```python
from build123d import *

# Parameters (mm, degrees)
F0_W     = 270
F0_H     = 32
F0_W_2   = 268
F0_H_2   = 30
F1_DEPTH = 210
F2_R     = 22.9
F3_DEPTH = 1
F4_R     = 1.5
F5_R     = 1


with BuildPart() as f1:
    # F0 (on Right) → F1 (new body)
    with BuildSketch(Plane.YZ):
        with Locations((135, -16)):
            Rectangle(F0_W, F0_H)
        with Locations((135, -16)):
            Rectangle(F0_W_2, F0_H_2, mode=Mode.SUBTRACT)
    extrude(amount=F1_DEPTH)

    # F2 (on face) → F3 (cut, through all)
    with BuildSketch(Plane.XY):
        with Locations((27.8, 29.6)):
            Circle(F2_R)
        with Locations((27.8, 82.6)):
            Circle(F2_R)
        with Locations((27.8, 135.6)):
            Circle(F2_R)
        with Locations((27.8, 188.6)):
            Circle(F2_R)
        with Locations((27.8, 241.6)):
            Circle(F2_R)
        with Locations((78.8, 29.6)):
            Circle(F2_R)
        with Locations((78.8, 82.6)):
            Circle(F2_R)
        with Locations((78.8, 135.6)):
            Circle(F2_R)
        with Locations((78.8, 188.6)):
            Circle(F2_R)
        with Locations((78.8, 241.6)):
            Circle(F2_R)
        with Locations((129.8, 29.6)):
            Circle(F2_R)
        with Locations((129.8, 82.6)):
            Circle(F2_R)
        with Locations((129.8, 135.6)):
            Circle(F2_R)
        with Locations((129.8, 188.6)):
            Circle(F2_R)
        with Locations((129.8, 241.6)):
            Circle(F2_R)
        with Locations((180.8, 29.6)):
            Circle(F2_R)
        with Locations((180.8, 82.6)):
            Circle(F2_R)
        with Locations((180.8, 135.6)):
            Circle(F2_R)
        with Locations((180.8, 188.6)):
            Circle(F2_R)
        with Locations((180.8, 241.6)):
            Circle(F2_R)
    extrude(amount=-F3_DEPTH, mode=Mode.SUBTRACT)

    # F4
    f4_edges = [f1.edges().sort_by_distance(p)[0] for p in [
        (105, 270, 0),
        (105, 270, -32),
        (105, 0, -32),
        (105, 0, 0),
    ]]
    fillet(f4_edges, radius=F4_R)

    # F5
    f5_edges = [f1.edges().sort_by_distance(p)[0] for p in [
        (105, 1, -1),
        (105, 1, -31),
        (105, 269, -31),
        (105, 269, -1),
    ]]
    fillet(f5_edges, radius=F5_R)


solid = f1.part
```
CAD build for the part. Positions are in the model's coordinates, mm. A direction names the side the tool comes from. Coordinates: 2 decimals unless noted, no trailing zeros. Order: outer loops, then holes, each group sorted by start corner. A loop starts at its lowest first (then second) coordinate and runs counter-clockwise, first axis right, second up. Notation, with made-up numbers: (35.25, 84.25) - (67.25, 84.25) arc R15 ccw to (67.25, 105.25) - close; hole circle Ø2 at (50.25, 2.25). An arc over 180 degrees is marked (long way). Answer in a Markdown table with one row per item.
1. Slice it at D-D, the plane y = 208.5. List the corners of the cut face in (x, z).
Answer:
| item | result |
|---|---|
| outline | (0, -32) - (210, -32) - (210, -31) - (0, -31) - close; (0, -1) - (16.47, -1) - (16.47, 0) - (0, 0) - close; (39.13, -1) - (67.47, -1) - (67.47, 0) - (39.13, 0) - close; (90.13, -1) - (118.47, -1) - (118.47, 0) - (90.13, 0) - close; (141.13, -1) - (169.47, -1) - (169.47, 0) - (141.13, 0) - close; (192.13, -1) - (210, -1) - (210, 0) - (192.13, 0) - close |
2. Slice it at B-B, the plane y = 241.6. List the corners of the cut face in (x, z).
Answer:
| item | result |
|---|---|
| outline | (0, -32) - (210, -32) - (210, -31) - (0, -31) - close; (0, -1) - (4.9, -1) - (4.9, 0) - (0, 0) - close; (50.7, -1) - (55.9, -1) - (55.9, 0) - (50.7, 0) - close; (101.7, -1) - (106.9, -1) - (106.9, 0) - (101.7, 0) - close; (152.7, -1) - (157.9, -1) - (157.9, 0) - (152.7, 0) - close; (203.7, -1) - (210, -1) - (210, 0) - (203.7, 0) - close |
3. Flat gauge pin, fed straight in: P1, Ø12, axis at x = 176, y = 97.5, coming from the +Z side. Where does the tip first touch, or does it go through?
Answer:
| item | result |
|---|---|
| P1 | z = -31 |
4. Slice it at C-C, the plane x = 78.8. Give the number of separate pieces and of enclosed holes in the cut face, then the cut area to 3 significant figures.
Answer:
| item | result |
|---|---|
| separate pieces | 5 |
| enclosed holes | 0 |
| area | 370 mm² |
5. Pull direction Y, two halves, no side cores. Call faces 4 (the face through (104, 133, -32)), 5 (the face through (104, 270, -16)), 6 (the face through (151.64, 89.48, -0.49)): +Y half, -Y half, draft (parallel to the pull), parting line (faces both ways), or undercut.
Answer:
| item | result |
|---|---|
| face 4 | draft |
| face 5 | +Y half |
| face 6 | undercut |
6. Slice it at A-A, the plane z = -5. List the corners of the cut face in (x, y), then the cut area to 3 significant figures.
Answer:
| item | result |
|---|---|
| outline | (0, 0) - (210, 0) - (210, 1) - (0, 1) - close; (0, 269) - (210, 269) - (210, 270) - (0, 270) - close |
| area | 420 mm² |
7. 3-axis set-ups, long thin cutter, end or side, ignore diameter. For faces 1 (the face through (104, 133, -1)), 2 (the face through (104, 0, -16)), 3 (the face through (142.11, 154.91, -0.49)): which of +Z, -Z, +X, -X, +Y, -Y reach the whole face in a straight line?
Answer:
| item | result |
|---|---|
| face 1 | +X, -X |
| face 2 | +Z, -Z, +X, -X, -Y |
| face 3 | +Z |
8. Drill centre lines: L1, parallel to Y at x = 61.5, z = -12.5; L2, parallel to Z at x = 61.5, y = 160; L3, parallel to Y at x = 78.8, z = -0.75. Where is each one in solid material? Low to high. Write a range as from..to.
Answer:
| item | result |
|---|---|
| L1 | 0..1, 269..270 |
| L2 | -32..-31, -1..0 |
| L3 | 0.2..6.7, 52.5..59.7, 105.5..112.7, 158.5..165.7, 211.5..218.7, 264.5..269.8 |
